```python
from build123d import *

# Parameters (mm, degrees)
SKETCH2_R           = 3
BOSS_EXTRUDE1_DEPTH = 18.1


with BuildPart() as part:
    # Sketch2 → Boss-Extrude1 (new body)
    with BuildSketch(Plane(origin=(0, 0, 0), x_dir=(1, 0, 0), z_dir=(0, 1, 0))):
        with BuildLine():
            Line((-191.397338403, -33.450570342), (21.552661597, -33.450570342))
            ThreePointArc((21.552661597, -33.450570342), (23.673981941, -32.571890686), (24.552661597, -30.450570342))
            Line((24.552661597, -30.450570342), (24.552661597, 62.524429658))
            Line((24.552661597, 62.524429658), (18.552661597, 62.524429658))
            Line((18.552661597, 62.524429658), (18.552661597, 74.524429658))
            Line((18.552661597, 74.524429658), (24.552661597, 74.524429658))
            Line((24.552661597, 74.524429658), (42.652661597, 74.524429658))
            Line((42.652661597, 74.524429658), (48.652661597, 74.524429658))
            Line((48.652661597, 74.524429658), (48.652661597, 62.524429658))
            Line((48.652661597, 62.524429658), (42.652661597, 62.524429658))
            Line((42.652661597, 62.524429658), (42.652661597, -30.450570342))
            ThreePointArc((42.652661597, -30.450570342), (43.531341253, -32.571890686), (45.652661597, -33.450570342))
            Line((45.652661597, -33.450570342), (258.602661597, -33.450570342))
            Line((258.602661597, -33.450570342), (42.652661597, 182.499429658))
            Line((42.652661597, 182.499429658), (24.552661597, 182.499429658))
            Line((24.552661597, 182.499429658), (-191.397338403, -33.450570342))
        make_face()
        with Locations((33.602661597, 170.499429658)):
            Circle(SKETCH2_R, mode=Mode.SUBTRACT)
        with Locations((235.716045652, -26.225419091)):
            Circle(SKETCH2_R, mode=Mode.SUBTRACT)
        with Locations((-168.510722458, -26.225419091)):
            Circle(SKETCH2_R, mode=Mode.SUBTRACT)
    extrude(amount=BOSS_EXTRUDE1_DEPTH)


solid = part.part
```
Geometry: final body of the model. Coordinates: model frame, mm. A direction names the side the tool comes from. Round coordinates to 2 decimals unless told otherwise and drop trailing zeros. Order: outer loops, then holes, each group sorted by start corner. A loop starts at its lowest first (then second) coordinate and runs counter-clockwise, first axis right, second up. Notation, with made-up numbers: (31.25, 19) -> (76.25, 19) arc R18 ccw to (76.25, 30) -> close; hole circle Ø4 at (56, -4). An arc over 180 degrees is marked (long way). Use one line per item in the form item = value. Start each with the question number.
1. Cut plane D-D (z = -30). Return the cut outline in (x, y).
2. Cut plane B-B (y = 9). Return the cut outline in (x, z).
3. Cut plane C-C (x = 85). Return the cut outline in (y, z).
4. Reachability of faces 1 (the face through (24.553, 9, -15)), 2 (the face through (48.653, 9, -69)), 3 (the face through (34, 9, -182.499)) from +Z, -Z, +X, -X, +Y, -Y: full face, straight path, thin tool, end or side. Return the list, or none.
5. Line query: probe 1 along X at (y, z) = (7.5, 13.5); probe 2 along X at (y, z) = (2.5, -42); probe 3 along X at (y, z) = (12.5, -118). Output: solid intervals per line, ascending.
6. Pin query (flat end, axial travel): pin 1 Ø4 at (x, y) = (-44.5, 14) entering from -Z; pin 2 Ø5.5 at (y, z) = (10, -34) entering from -X; pin 3 Ø5.5 at (y, z) = (6, 1) entering from +X. Return the tip coordinate at first contact, or that it passes through.
7. Draft query along Z for faces 4 (the face through (33, 9, -74.524)), 5 (the face through (152.14, 8.92, -73.01)), 6 (the face through (30, 18.1, -76)), 7 (the face through (18.553, 9, -68)). Return one class per face: pulls with the +Z half, pulls with the -Z half, needs draft (parallel to the pull), parting line crosses it, or undercut.
8. Cut plane A-A (z = 14). Return the cut outline in (x, y).
Solution:
q1.outline = (-127.95, 0) -> (24.55, 0) -> (24.55, 18.1) -> (-127.95, 18.1) -> close; (42.65, 0) -> (195.15, 0) -> (195.15, 18.1) -> (42.65, 18.1) -> close
q2.outline = (-191.4, 33.45) -> (24.55, -182.5) -> (42.65, -182.5) -> (258.6, 33.45) -> (45.65, 33.45) arc R3 ccw to (42.65, 30.45) -> (42.65, -62.52) -> (48.65, -62.52) -> (48.65, -74.52) -> (18.55, -74.52) -> (18.55, -62.52) -> (24.55, -62.52) -> (24.55, 30.45) arc R3 ccw to (21.55, 33.45) -> close; hole circle Ø6 at (-168.51, 26.23); hole circle Ø6 at (33.6, -170.5); hole circle Ø6 at (235.72, 26.23)
q3.outline = (0, -140.15) -> (18.1, -140.15) -> (18.1, 33.45) -> (0, 33.45) -> close
q4.face_1 = +Z, +Y, -Y
q4.face_2 = +Y, -Y
q4.face_3 = -Z, +X, -X, +Y, -Y
q5.probe_1 = -171.45 to 24.55, 42.65 to 238.65
q5.probe_2 = -115.95 to 24.55, 42.65 to 183.15
q5.probe_3 = -39.95 to 107.15
q6.pin_1 = -115.45
q6.pin_2 = -126.7
q6.pin_3 = 228.9
q7.face_4 = undercut
q7.face_5 = pulls with the -Z half
q7.face_6 = needs draft
q7.face_7 = undercut
q8.outline = (-171.95, 0) -> (24.55, 0) -> (24.55, 18.1) -> (-171.95, 18.1) -> close; (42.65, 0) -> (239.15, 0) -> (239.15, 18.1) -> (42.65, 18.1) -> close
